```python
from build123d import *

# Parameters (mm, degrees)
EXTRUIR1_DEPTH = 0.5
EXTRUIR2_DEPTH = 135.945083127
CROQUIS3_W     = 7.84225
CROQUIS3_H     = 7.7
CROQUIS3_W_2   = 13
CROQUIS3_H_2   = 43
CROQUIS3_W_3   = 8
CROQUIS3_H_3   = 5
CROQUIS3_W_4   = 5
CROQUIS3_H_4   = 41.175
EXTRUIR3_DEPTH = 0.1


with BuildPart() as part:
    # Croquis1 → Extruir1 (new, symmetric)
    with BuildSketch(Plane(origin=(0, 0, 0), x_dir=(1, 0, 0), z_dir=(0, 1, 0))):
        Polygon((7.84225, -38.65625), (7.84225, -32.54375), (0, -32.54375), (0, 32.54375), (7.84225, 32.54375), (7.84225, 37.54375), (124.5235, 37.54375), (124.5235, 33.3375), (129.286, 33.3375), (129.286, -33.3375), (124.5235, -33.3375), (124.5235, -38.65625), align=None)
    extrude(amount=EXTRUIR1_DEPTH, both=True)

    # Croquis2 → Extruir2 (cut, through all)
    with BuildSketch(Plane(origin=(0, 0.5, 0), x_dir=(1, 0, 0), z_dir=(0, 1, 0))):
        with BuildLine():
            Line((30, 32.4), (42, 32.4))
            ThreePointArc((42, 32.4), (43.5, 30.9), (42, 29.4))
            Line((42, 29.4), (30, 29.4))
            ThreePointArc((30, 29.4), (28.5, 30.9), (30, 32.4))
        make_face()
        with BuildLine():
            Line((109.786, 32.4), (121.786, 32.4))
            ThreePointArc((121.786, 32.4), (123.286, 30.9), (121.786, 29.4))
            Line((121.786, 29.4), (109.786, 29.4))
            ThreePointArc((109.786, 29.4), (108.286, 30.9), (109.786, 32.4))
        make_face()
    extruir2 = extrude(amount=-EXTRUIR2_DEPTH, mode=Mode.SUBTRACT)

    # Simetría1: Extruir2 across plane
    add(extruir2.mirror(Plane.XY), mode=Mode.SUBTRACT)

    # Croquis3 → Extruir3 (add)
    with BuildSketch(Plane(origin=(0, 0.5, 0), x_dir=(1, 0, 0), z_dir=(0, 1, 0))):
        with Locations((3.921125, 0.1124)):
            Rectangle(CROQUIS3_W, CROQUIS3_H)
        with Locations((19.5, 3.04375)):
            Rectangle(CROQUIS3_W_2, CROQUIS3_H_2)
        with Locations((4, 23.93125)):
            Rectangle(CROQUIS3_W_3, CROQUIS3_H_3)
        with Locations((125.786, -4.5)):
            Rectangle(CROQUIS3_W_4, CROQUIS3_H_4)
    extrude(amount=EXTRUIR3_DEPTH)


solid = part.part
```
Can you work these out from the model? Positions are in its coordinate system, mm. Coordinates: 2 decimals unless noted, no trailing zeros. Loops run counter-clockwise (first coordinate to the right, second up) from the corner with the lowest first, then second, coordinate; pieces in that order, holes last. Notation, with made-up numbers: (38, 62) - (85, 62) arc R17 cw to (85, 80) - close; hole circle Ø10 at (79, 51). An arc over 180 degrees is marked (long way). Use a Markdown table: item, result.
Item 1: I want a section at D-D on z = 0. Please give me the cut outline in (x, y), and give its area (3 significant figures).
Numbers:
| item | result |
|---|---|
| outline | (0, -0.5) - (129.29, -0.5) - (129.29, 0.5) - (128.29, 0.5) - (128.29, 0.6) - (123.29, 0.6) - (123.29, 0.5) - (26, 0.5) - (26, 0.6) - (13, 0.6) - (13, 0.5) - (7.84, 0.5) - (7.84, 0.6) - (0, 0.6) - close |
| area | 132 mm2 |
Item 2: We'd pull the mould along X, two halves only. Please class faces 1 (the face through (66, 0.5, 0)), 2 (the face through (19, 0.6, -3)): released by +X, released by -X, zero draft, split by the parting line, or undercut.
Numbers:
| item | result |
|---|---|
| face 1 | undercut |
| face 2 | zero draft |
Item 3: If I drill on probe 1 along Z at (x, y) = (36, 0.45); probe 2 along X at (y, z) = (-0.4, -31.5); probe 3 along X at (y, z) = (0.55, -4), over which ranges is the centre line in solid material (lowest first)? Write a range as from..to.
Numbers:
| item | result |
|---|---|
| probe 1 | z = -37.54..-32.4, -29.4..29.4, 32.4..38.66 |
| probe 2 | x = 0..28.63, 43.37..108.41, 123.16..129.29 |
| probe 3 | x = 13..26, 123.29..128.29 |
Item 4: I want a section at A-A on z = -30.9. Please give me the cut outline in (x, y).
Numbers:
| item | result |
|---|---|
| outline | (0, -0.5) - (28.5, -0.5) - (28.5, 0.5) - (0, 0.5) - close; (43.5, -0.5) - (108.29, -0.5) - (108.29, 0.5) - (43.5, 0.5) - close; (123.29, -0.5) - (129.29, -0.5) - (129.29, 0.5) - (123.29, 0.5) - close |
Item 5: I want a section at B-B on x = 35. Please give me the cut outline in (y, z).
Numbers:
| item | result |
|---|---|
| outline | (-0.5, -37.54) - (0.5, -37.54) - (0.5, -32.4) - (-0.5, -32.4) - close; (-0.5, -29.4) - (0.5, -29.4) - (0.5, 29.4) - (-0.5, 29.4) - close; (-0.5, 32.4) - (0.5, 32.4) - (0.5, 38.66) - (-0.5, 38.66) - close |
Item 6: Will these pins go through, and if not, where does the flat tip stop? pin 1 (10 mm diameter, centred on x = 69.5, z = -21, fed in from +Y); pin 2 (0.5 mm diameter, centred on y = 0, z = 34.5, fed in from -X).
Numbers:
| item | result |
|---|---|
| pin 1 | stops at y = 0.5 |
| pin 2 | stops at x = 7.84 |
Item 7: I want a section at C-C on y = 0.3. Please give me the cut outline in (x, z).
Numbers:
| item | result |
|---|---|
| outline | (0, -32.54) - (7.84, -32.54) - (7.84, -37.54) - (124.52, -37.54) - (124.52, -33.34) - (129.29, -33.34) - (129.29, 33.34) - (124.52, 33.34) - (124.52, 38.66) - (7.84, 38.66) - (7.84, 32.54) - (0, 32.54) - close; hole (30, -32.4) - (42, -32.4) arc R1.5 ccw to (42, -29.4) - (30, -29.4) arc R1.5 ccw to start; hole (30, 29.4) - (42, 29.4) arc R1.5 ccw to (42, 32.4) - (30, 32.4) arc R1.5 ccw to start; hole (109.79, -32.4) - (121.79, -32.4) arc R1.5 ccw to (121.79, -29.4) - (109.79, -29.4) arc R1.5 ccw to start; hole (109.79, 29.4) - (121.79, 29.4) arc R1.5 ccw to (121.79, 32.4) - (109.79, 32.4) arc R1.5 ccw to start |
